The listing builds one solid part. Answer for the finished solid, in the listing's coordinates (mm). A direction names the side the tool comes from. Give positions to 0.01 mm unless a question says otherwise; leave off trailing zeros. Loops run counter-clockwise (first coordinate to the right, second up) from the corner with the lowest first, then second, coordinate; pieces in that order, holes last. Notation, with made-up numbers: M 76,51.5 L 131,51.5 A19 ccw 131,68.5 Z; hole C -32.5,70 d3. An arc over 180 degrees is marked long. Return JSON: item names as keys, results as strings.
from build123d import *

# Parameters (mm, degrees)
BOSS_EXTRUDE1_DEPTH = 216
SKETCH3_W           = 240.4
SKETCH3_H           = 260
BOSS_EXTRUDE2_DEPTH = 8
SKETCH4_R           = 100
CUT_EXTRUDE1_DEPTH  = 8
CUT_EXTRUDE1_DRAFT  = -42.88487357
SKETCH6_W           = 240.4
SKETCH6_H           = 208
BOSS_EXTRUDE3_DEPTH = 8
SKETCH7_R           = 64.93911957
CUT_EXTRUDE2_DEPTH  = 8
CUT_EXTRUDE2_DRAFT  = -42.88487357
SKETCH8_W           = 70.3
SKETCH8_H           = 200
CUT_EXTRUDE3_DEPTH  = 8
SKETCH9_W           = 256.4
SKETCH9_H           = 216
SKETCH9_W_2         = 240.4
SKETCH9_H_2         = 200
BOSS_EXTRUDE4_DEPTH = 35.2
SKETCH12_W          = 240.4
SKETCH12_H          = 153.003510621
BOSS_EXTRUDE6_DEPTH = 8
SKETCH13_W          = 64.11038507
SKETCH13_H          = 150
CUT_EXTRUDE6_DEPTH  = 8
SKETCH15_W          = 49.9
SKETCH15_H          = 184
CUT_EXTRUDE8_DEPTH  = 8
SKETCH16_W          = 70.2
SKETCH16_H          = 8
SKETCH16_W_2        = 70.1
BOSS_EXTRUDE7_DEPTH = 8
SKETCH19_W          = 15
SKETCH19_H          = 106.796489379
BOSS_EXTRUDE8_DEPTH = 8
FILLET2_R           = 8
FILLET3_R           = 2
FILLET4_R           = 2
FILLET5_R           = 2
SKETCH20_W          = 29
SKETCH20_H          = 30
CUT_EXTRUDE9_DEPTH  = 10
FILLET6_R           = 2


with BuildPart() as part:
    # Sketch2 → Boss-Extrude1 (new body)
    with BuildSketch(Plane(origin=(0, 0, 0), x_dir=(1, 0, 0), z_dir=(0, 1, 0))):
        Polygon((256.4, 0), (248.4, 0), (248.4, 260), (8, 260), (8, 0), (0, 0), (0, 268), (256.4, 268), align=None)
    extrude(amount=BOSS_EXTRUDE1_DEPTH)

    # Sketch3 → Boss-Extrude2 (add)
    with BuildSketch(Plane.XZ):
        with Locations((128.2, -130)):
            Rectangle(SKETCH3_W, SKETCH3_H)
    extrude(amount=-BOSS_EXTRUDE2_DEPTH)


with BuildPart() as cut_extrude1_tool:
    # Sketch4 → Cut-Extrude1 (with draft: the straight prism first)
    with BuildSketch(Plane(origin=(0, 0, -268), x_dir=(-1, 0, 0), z_dir=(0, 0, -1))):
        with Locations((-128.2, 108)):
            Circle(SKETCH4_R)
    extrude(amount=-CUT_EXTRUDE1_DEPTH)
    # Cut-Extrude1: the draft: its side faces are tilted about the plane it starts from
    cut_extrude1_sides = [cut_extrude1_tool.faces().sort_by_distance(p)[0] for p in [
        (228.2, 108, -264),
    ]]
    draft(cut_extrude1_sides, Plane(origin=(0, 0, -268), x_dir=(-1, 0, 0), z_dir=(0, 0, -1)), CUT_EXTRUDE1_DRAFT)


with BuildPart() as part_1:
    add(part.part)

    # Cut-Extrude1: cut by cut_extrude1_tool
    add(cut_extrude1_tool.part, mode=Mode.SUBTRACT)

    # Sketch6 → Boss-Extrude3 (add)
    with BuildSketch(Plane.XY.offset(-230.3)):
        with Locations((128.2, 112)):
            Rectangle(SKETCH6_W, SKETCH6_H)
    extrude(amount=BOSS_EXTRUDE3_DEPTH)


with BuildPart() as cut_extrude2_tool:
    # Sketch7 → Cut-Extrude2 (with draft: the straight prism first)
    with BuildSketch(Plane(origin=(0, 0, -230.3), x_dir=(-1, 0, 0), z_dir=(0, 0, -1))):
        with Locations((-128.2, 108)):
            Circle(SKETCH7_R)
    extrude(amount=-CUT_EXTRUDE2_DEPTH)
    # Cut-Extrude2: the draft: its side faces are tilted about the plane it starts from
    cut_extrude2_sides = [cut_extrude2_tool.faces().sort_by_distance(p)[0] for p in [
        (193.13911957, 108, -226.3),
    ]]
    draft(cut_extrude2_sides, Plane(origin=(0, 0, -230.3), x_dir=(-1, 0, 0), z_dir=(0, 0, -1)), CUT_EXTRUDE2_DRAFT)


with BuildPart() as part_2:
    add(part_1.part)

    # Cut-Extrude2: cut by cut_extrude2_tool
    add(cut_extrude2_tool.part, mode=Mode.SUBTRACT)

    # Sketch8 → Cut-Extrude3 (cut)
    with BuildSketch(Plane.ZY):
        with Locations((-35.15, 108)):
            Rectangle(SKETCH8_W, SKETCH8_H)
    extrude(amount=-CUT_EXTRUDE3_DEPTH, mode=Mode.SUBTRACT)

    # Sketch9 → Boss-Extrude4 (add)
    with BuildSketch(Plane.XY.offset(35)):
        with Locations((128.2, 108)):
            Rectangle(SKETCH9_W, SKETCH9_H)
        with Locations((128.2, 108)):
            Rectangle(SKETCH9_W_2, SKETCH9_H_2, mode=Mode.SUBTRACT)
    extrude(amount=-BOSS_EXTRUDE4_DEPTH)

    # Sketch12 → Boss-Extrude6 (add)
    with BuildSketch(Plane(origin=(0, 216, 0), x_dir=(1, 0, 0), z_dir=(0, 1, 0))):
        with Locations((128.2, 76.701755311)):
            Rectangle(SKETCH12_W, SKETCH12_H)
    extrude(amount=-BOSS_EXTRUDE6_DEPTH)

    # Sketch13 → Cut-Extrude6 (cut)
    with BuildSketch(Plane(origin=(256.4, 0, 0), x_dir=(0, 0, -1), z_dir=(1, 0, 0))):
        with Locations((32.055192535, 107.5)):
            Rectangle(SKETCH13_W, SKETCH13_H)
    extrude(amount=-CUT_EXTRUDE6_DEPTH, mode=Mode.SUBTRACT)

    # Sketch15 → Cut-Extrude8 (cut)
    with BuildSketch(Plane.ZY):
        with Locations((-95.25, 108)):
            Rectangle(SKETCH15_W, SKETCH15_H)
    extrude(amount=-CUT_EXTRUDE8_DEPTH, mode=Mode.SUBTRACT)

    # Sketch16 → Boss-Extrude7 (add)
    with BuildSketch(Plane.ZY):
        with Locations((-35.2, 12)):
            Rectangle(SKETCH16_W, SKETCH16_H)
        with Locations((-35.25, 204)):
            Rectangle(SKETCH16_W_2, SKETCH16_H)
    extrude(amount=-BOSS_EXTRUDE7_DEPTH)

    # Sketch19 → Boss-Extrude8 (add)
    with BuildSketch(Plane(origin=(0, 216, 0), x_dir=(1, 0, 0), z_dir=(0, 1, 0))):
        with Locations((15.5, 206.601755311)):
            Rectangle(SKETCH19_W, SKETCH19_H)
        with Locations((240.9, 206.601755311)):
            Rectangle(SKETCH19_W, SKETCH19_H)
    extrude(amount=-BOSS_EXTRUDE8_DEPTH)

    # Fillet2
    fillet2_edges = [part_2.edges().sort_by_distance(p)[0] for p in [
        (0, 0, -116.5),
        (0, 108, -268),
        (256.4, 108, -268),
        (256.4, 216, -116.5),
        (128.2, 216, -268),
        (0, 216, -116.5),
        (128.2, 0, -268),
        (256.4, 0, -116.5),
    ]]
    fillet(fillet2_edges, radius=FILLET2_R - 0.0001)  # a hair under: the kernel refuses the full size

    # Fillet3
    fillet3_edges = [part_2.edges().sort_by_distance(p)[0] for p in [
        (8, 208, -93.65),
        (248.4, 208, -93.65),
        (248.4, 8, -93.65),
        (8, 8, -93.65),
    ]]
    fillet(fillet3_edges, radius=FILLET3_R)

    # Fillet4
    fillet4_edges = [part_2.edges().sort_by_distance(p)[0] for p in [
        (16.5, 208, -222.3),
        (239.9, 208, -222.3),
        (248.4, 108, -222.3),
        (128.2, 8, -222.3),
        (8, 108, -222.3),
        (8.585786438, 207.414213562, -222.3),
        (247.814213562, 207.414213562, -222.3),
        (8.585786438, 8.585786438, -222.3),
        (247.814213562, 8.585786438, -222.3),
    ]]
    fillet(fillet4_edges, radius=FILLET4_R)

    # Fillet5
    fillet5_edges = [part_2.edges().sort_by_distance(p)[0] for p in [
        (252.4, 32.5, 0),
        (252.4, 182.5, 0),
        (252.4, 182.5, -64.11038507),
        (252.4, 32.5, -64.11038507),
        (4, 16, -120.2),
        (4, 200, -120.2),
        (4, 16, -0.2),
        (4, 200, -0.2),
    ]]
    fillet(fillet5_edges, radius=FILLET5_R)

    # Sketch20 → Cut-Extrude9 (cut)
    with BuildSketch(Plane.ZY):
        with Locations((-166.055192535, 107.75)):
            Rectangle(SKETCH20_W, SKETCH20_H)
    extrude(amount=-CUT_EXTRUDE9_DEPTH, mode=Mode.SUBTRACT)

    # Fillet6
    fillet6_edges = [part_2.edges().sort_by_distance(p)[0] for p in [
        (4, 122.75, -151.555192535),
        (4, 92.75, -151.555192535),
        (4, 92.75, -180.555192535),
        (4, 122.75, -180.555192535),
    ]]
    fillet(fillet6_edges, radius=FILLET6_R)


solid = part_2.part
(1) Determine the mould class of faces 1 (the flat face through (256.4, 107, -143)), 2 (the flat face through (4, 108, -180.555)), 3 (the flat face through (127, 8, -91)) for opening direction X: released by +X, released by -X, zero draft, split by the parting line, or undercut.
Values follow:
{"face 1": "released by +X", "face 2": "zero draft", "face 3": "undercut"}
(2) Given pin 1 (1.5 mm diameter, centred on x = 76.5, y = 135.5, fed in from +Z); pin 2 (2.5 mm diameter, centred on y = 210, z = -251, fed in from -X); pin 3 (9 mm diameter, centred on x = 253.5, y = 73.5, fed in from -Z), each flat-ended and moving along its own axis, determine where each tip first touches the part or whether it passes through.
Values follow:
{"pin 1": "z = -222.3", "pin 2": "x = 0.04", "pin 3": "z = -267.98"}
(3) Straight lines are drawn through the part: line 1 along Z through (x, y) = (239.5, 147.5); line 2 along X through (y, z) = (33, -205); line 3 along Y through (x, z) = (30, -141). For each, find the intervals that lie inside material, in ascending order.
Values follow:
{"line 1": "-268 to -260, -230.3 to -222.3", "line 2": "0 to 8, 248.4 to 256.4", "line 3": "0 to 8, 208 to 216"}
(4) The part is cut by section A-A (z = -46.5). Determine the outline of the cut face in (x, y), and give its area (3 significant figures).
Values follow:
{"outline": "M 0,8 A8 ccw 8,0 L 248.4,0 A8 ccw 256.4,8 L 256.4,32.5 L 248.4,32.5 L 248.4,10 A2 cw 246.4,8 L 10,8 A2 cw 8,10 L 8,16 L 0,16 Z; M 0,200 L 8,200 L 8,206 A2 cw 10,208 L 246.4,208 A2 cw 248.4,206 L 248.4,182.5 L 256.4,182.5 L 256.4,208 A8 ccw 248.4,216 L 8,216 A8 ccw 0,208 Z", "area": "4,580 mm²"}
(5) The part is cut by section B-B (x = 128.2). Give the number of separate pieces and of enclosed holes in the cut face, and give its area (3 significant figures).
Values follow:
{"separate pieces": "4", "enclosed holes": "0", "area": "4,710 mm²"}
(6) A tool of negligible diameter and unlimited length cuts with its end or side. For faces 4 (the flat face through (118, 5, 35)), 5 (the flat face through (252, 182.5, -32)), 6 (the flat face through (233.4, 212, -245)), 7 (the flat face through (8, 107, -245)), from which of +Z, -Z, +X, -X, +Y, -Y can it reach the whole face along a straight path? Write none if from no direction.
Values follow:
{"face 4": "+Z, +X, -X, +Y, -Y", "face 5": "+X, -X", "face 6": "+Y", "face 7": "none"}
(7) The part is cut by section C-C (z = -188). Determine the outline of the cut face in (x, y), and give its area (3 significant figures).
Values follow:
{"outline": "M 0,8 A8 ccw 8,0 L 248.4,0 A8 ccw 256.4,8 L 256.4,208 A8 ccw 248.4,216 L 233.4,216 L 233.4,208 L 246.4,208 A2 cw 248.4,206 L 248.4,10 A2 cw 246.4,8 L 10,8 A2 cw 8,10 L 8,206 A2 cw 10,208 L 23,208 L 23,216 L 8,216 A8 ccw 0,208 Z", "area": "5,570 mm²"}
